```python
from build123d import *

# Parameters (mm, degrees)
F1_FACE_R = 78.866989
F2_DEPTH  = 25.4


with BuildPart() as f1:
    # F0 (on Front) → F1 (revolve)
    with BuildSketch(Plane.XZ):
        Polygon((0, -254), (0, -19.925557), (-78.866989, -19.925557), (-85.947688, -70.212811), (-85.947688, -197.212811), (-86.925529, -198.023198), (-86.925529, -223.423198), (-78.866989, -227.221664), (-86.925529, -230.975599), (-76.2, -254), align=None)
    revolve(axis=Axis((0, 0, -127), (0, 0, -1)))

    # F1_face (on face) → F2 (join)
    with BuildSketch(Plane.XY.offset(-19.925557)):
        Circle(F1_FACE_R)
    extrude(amount=F2_DEPTH)


solid = f1.part
```
For this review, take the finished solid that the model builds, in its own axes (mm). A direction names the side the tool comes from. Coordinates: 2 decimals unless noted, no trailing zeros. Loops run counter-clockwise (first coordinate to the right, second up) from the corner with the lowest first, then second, coordinate; pieces in that order, holes last.
1. Add section A-A, the plane y = 0. Give the boundary of the cut face in (x, z), then the cut area to 3 significant figures.
2. For faces 1 (the flat face through (-1, 1, 5.474)), 2 (the cylindrical face through (-10.267, 78.196, -7.403)), 3 (the conical face through (10.33, 78.7, -227.46)), list the 3-axis set-ups (+Z, -Z, +X, -X, +Y, -Y) from which the entire face can be reached by the end or side of a thin tool; tool diameter is ignored.
3. For line 1 (Y direction, x = -3, z = -118.5); line 2 (Z direction, x = -60, y = -62); line 3 (Z direction, x = 28, y = 72), list the stretches that pass through material, from the lowest coordinate up.
4. Mouldability with a two-part tool opening along Z and no side actions: class faces 4 (the conical face through (-37.32, -71.76, -34.25)), 5 (the conical face through (-73.21, -30.36, -227.04)), 6 (the cylindrical face through (18.84, -84.86, -210.9)) as +Z half, -Z half, draft (parallel to the pull), parting line (faces both ways), or undercut.
5. Add section D-D, the plane z = -236. Give the boundary of the cut face in (x, y) (3 decimals).
6. Insertion check: P1, Ø6, axis at x = 10.5, z = -209.5, coming from the -Y side; P2, Ø1.5, axis at x = -67, z = -186.5, coming from the -Y side; P3, Ø10, axis at x = 61, z = -90, coming from the +Y side. Each pin has a flat end and moves straight along its axis. Give the tip position at first contact, or say it passes through.
7. Add section C-C, the plane z = -188. Give the boundary of the cut face in (x, y), then the cut area to 3 significant figures.
Result:
1. outline: (-86.93, -230.98) - (-76.2, -254) - (76.2, -254) - (86.93, -230.98) - (78.87, -227.22) - (86.93, -223.42) - (86.93, -198.02) - (85.95, -197.21) - (85.95, -70.21) - (78.87, -19.93) - (78.87, 5.47) - (-78.87, 5.47) - (-78.87, -19.93) - (-85.95, -70.21) - (-85.95, -197.21) - (-86.93, -198.02) - (-86.93, -223.42) - (-78.87, -227.22) - close
1. area: 43,700 mm2
2. face 1: +Z, +X, -X, +Y, -Y
2. face 2: +Z
2. face 3: none
3. line 1: y = -85.9 to 85.9
3. line 2: z = -232.36 to -230.67, -223.73 to -197.49
3. line 3: z = -251.74 to 5.47
4. face 4: +Z half
4. face 5: undercut
4. face 6: draft
5. outline: circle Ø169.17 at (0, 0)
6. P1: stops at y = -86.6
6. P2: stops at y = -54.75
6. P3: stops at y = 65.2
7. outline: circle Ø171.9 at (0, 0)
7. area: 23,200 mm2
